Source: CAD feature listing. Evaluate the final solid. Frame: model axes, mm. Face numbers are marked on the shaded views. Round coordinates to 2 decimals unless told otherwise and drop trailing zeros. Order: outer loops, then holes, each group sorted by start corner. A loop starts at its lowest first (then second) coordinate and runs counter-clockwise, first axis right, second up. Notation, with made-up numbers: M 39,-26.5 L 43,-26.5 A33 cw 43,3.5 Z; hole C 29.25,4 d2. An arc over 180 degrees is marked long. Use one line per item in the form item = value. Start each with the question number.
Q1. Section B-B (z = -7.5). Return the cut outline in (x, y), plus the area to 3 significant figures.
Q2. Pull-direction query (Z, two-part tool) for the marked faces 1, 2 and 3; classes: pulls with the +Z half, pulls with the -Z half, needs draft (parallel to the pull), parting line crosses it, or undercut.
Q3. Contact query for flat-ended pins moving along their axis: pin 1 (1 mm diameter, centred on x = 96.5, y = 12.5, fed in from +Z); pin 2 (1 mm diameter, centred on y = 11.5, z = -6.5, fed in from +X); pin 3 (2 mm diameter, centred on y = 7, z = -8.5, fed in from -X). Output: stop coordinate, or through.
Q4. Material intervals for probe 1 along X at (y, z) = (4, -8.75); probe 2 along X at (y, z) = (12.75, -8.75); probe 3 along Y at (x, z) = (97, -11), sorted ascending.
Q5. Section A-A (x = 95.75). Return the cut outline in (y, z).
Q6. Section C-C (y = 14). Return the cut outline in (x, z), plus the area to 3 significant figures.
Q7. Section D-D (y = 7). Return the cut outline in (x, z), plus the area to 3 significant figures.
from build123d import *

# Parameters (mm, degrees)
SKETCH_2_R          = 3.5
SKETCH_2_R_2        = 1.65
EXTRUDE_1_DEPTH     = 1
SKETCH_3_R          = 2.2
EXTRUDE_2_DEPTH     = 20
SKETCH_6_R          = 1.65
CUT_EXTRUDE_1_DEPTH = 10


with BuildPart() as part:
    # 草图2 → 凸台-拉伸1 (new body)
    with BuildSketch(Plane.XZ):
        with Locations((96.952704723, -8.683144071)):
            Circle(SKETCH_2_R)
        with Locations((96.952704723, -8.683144071)):
            Circle(SKETCH_2_R_2, mode=Mode.SUBTRACT)
    extrude(amount=EXTRUDE_1_DEPTH)

    # 草图3 → 凸台-拉伸2 (add)
    with BuildSketch(Plane(origin=(0, 0, 0), x_dir=(1, 0, 0), z_dir=(0, 1, 0))):
        with Locations((96.952704723, 8.683144071)):
            Circle(SKETCH_3_R)
    extrude(amount=EXTRUDE_2_DEPTH)

    # 草图6 → 切除-拉伸1 (cut)
    with BuildSketch(Plane.XZ):
        with Locations((96.952704723, -8.683144071)):
            Circle(SKETCH_6_R)
    extrude(amount=-CUT_EXTRUDE_1_DEPTH, mode=Mode.SUBTRACT)


solid = part.part
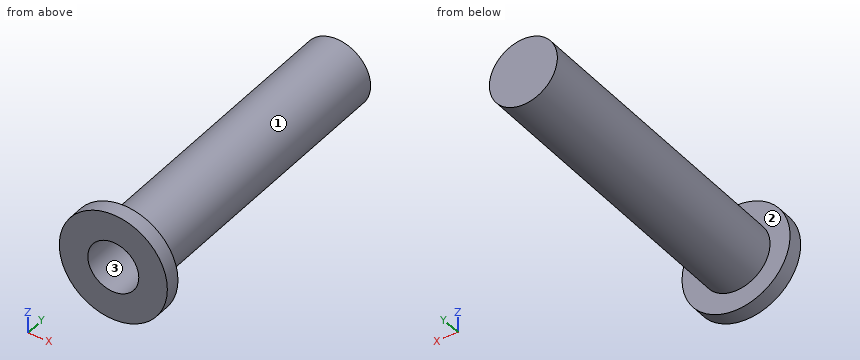
Results list:
q1.outline = M 93.66,-1 L 95.8,-1 L 95.8,10 L 98.1,10 L 98.1,-1 L 100.25,-1 L 100.25,0 L 98.81,0 L 98.81,20 L 95.1,20 L 95.1,0 L 93.66,0 Z
q1.area = 55.5 mm2
q2.face_1 = parting line crosses it
q2.face_2 = needs draft
q2.face_3 = undercut
q3.pin_1 = -6.48
q3.pin_2 = 98.37
q3.pin_3 = 94.75
q4.probe_1 = 94.75 to 95.3, 98.6 to 99.15
q4.probe_2 = 94.75 to 99.15
q4.probe_3 = -1 to 0
q5.outline = M -1,-11.97 L 0,-11.97 L 0,-10.53 L 20,-10.53 L 20,-6.84 L 0,-6.84 L 0,-5.4 L -1,-5.4 L -1,-7.55 L 10,-7.55 L 10,-9.81 L -1,-9.81 Z
q6.outline = C 96.95,-8.68 d4.4
q6.area = 15.2 mm2
q7.outline = C 96.95,-8.68 d4.4; hole C 96.95,-8.68 d3.3
q7.area = 6.65 mm2
